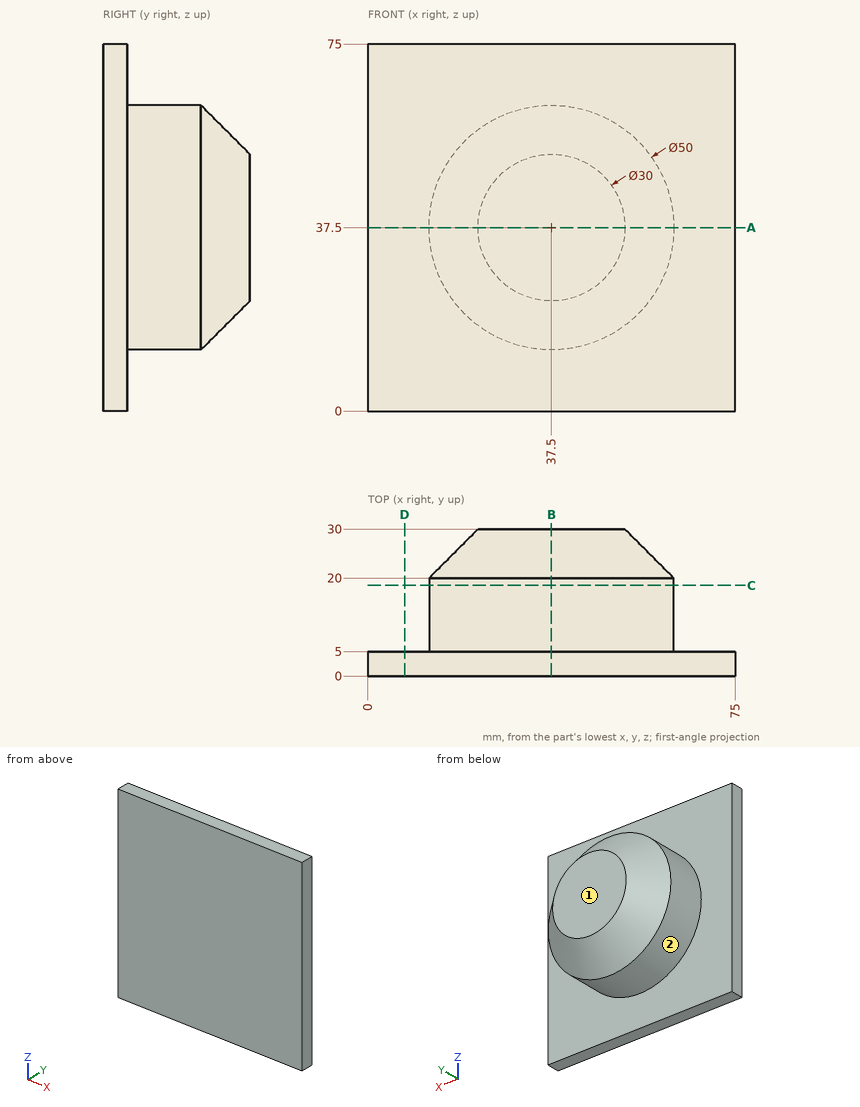
Part print with two shaded views. Sizes in mm from the minimum x, y, z corner. A direction names the side the tool comes from. Coordinates: 2 decimals unless noted, no trailing zeros. Write each loop counter-clockwise with the first axis right and the second up, starting at its lowest first coordinate (ties: lowest second). Pieces come first, ordered by that corner, then holes. Notation, with made-up numbers: (15.5, 63.25) - (44.5, 63.25) arc R17 cw to (44.5, 88.25) - close; hole circle Ø11 at (-33, -27.5). An arc over 180 degrees is marked (long way). One line per item, written item: value. Start each with the question number.
1. Slice it at B-B (x = 37.5). Write the cut outline in (y, z).
2. Flat gauge pins, fed straight in: pin 1 (1.5 mm diameter, centred on x = 24, z = 17.5, fed in from +Y); pin 2 (8 mm diameter, centred on y = 21, z = 33, fed in from +X); pin 3 (1.5 mm diameter, centred on y = 26.5, z = 39.5, fed in from +X); pin 4 (12 mm diameter, centred on y = 26, z = 65.5, fed in from +X). Where does each tip first touch, or does it go through?
3. Slice it at C-C (y = 18.5). Write the cut outline in (x, z).
4. Tool access for the marked faces 1 and 2: list every direction of +Z, -Z, +X, -X, +Y, -Y with a clear straight run to the whole face (end or side of a thin tool).
5. Slice it at D-D (x = 7.5). Write the cut outline in (y, z).
6. Probe line 1 (Y direction, x = 6.5, z = 51); line 2 (Y direction, x = 35.5, z = 18); line 3 (Z direction, x = 20.5, y = 9.5). List the from-to ranges inside material, lowest first. Write a range as from..to.
7. Slice it at A-A (z = 37.5). Write the cut outline in (x, y).
Answers below:
1. outline: (0, 0) - (5, 0) - (5, 12.5) - (20, 12.5) - (30, 22.5) - (30, 52.5) - (20, 62.5) - (5, 62.5) - (5, 75) - (0, 75) - close
2. pin 1: stops at y = 21.62
2. pin 2: stops at x = 62.49
2. pin 3: stops at x = 56.65
2. pin 4: passes through
3. outline: circle Ø50 at (37.5, 37.5)
4. face 1: +Z, -Z, +X, -X, +Y
4. face 2: +Y
5. outline: (0, 0) - (5, 0) - (5, 75) - (0, 75) - close
6. line 1: y = 0..5
6. line 2: y = 0..25.4
6. line 3: z = 19.17..55.83
7. outline: (0, 0) - (75, 0) - (75, 5) - (62.5, 5) - (62.5, 20) - (52.5, 30) - (22.5, 30) - (12.5, 20) - (12.5, 5) - (0, 5) - close
